Answer from the drawing. Dimensions are ordinates in mm from the lowest x, y and z of the part. A direction names the side the tool comes from. Coordinates: 2 decimals unless noted, no trailing zeros. Write each loop counter-clockwise with the first axis right and the second up, starting at its lowest first coordinate (ties: lowest second). Pieces come first, ordered by that corner, then holes.
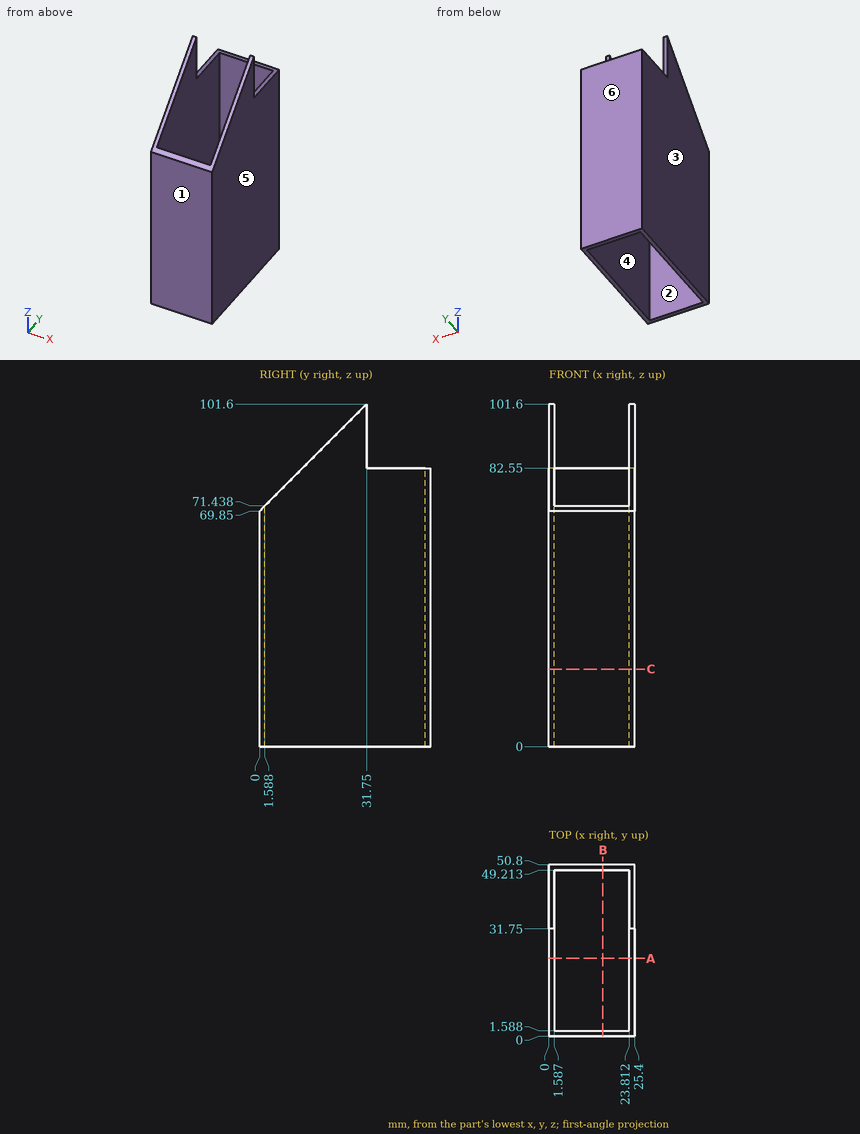
(1) This flat-tipped pin is pushed along its axis until it touches: pin 1 (0.5 mm diameter, centred on x = 25, z = 89.5, fed in from +Y). Where does it stop, or does it pass through?
(2) Which of the six approach directions +Z, -Z, +X, -X, +Y, -Y give full straight-line access (tool end or side, diameter ignored) to the marked faces 1 and 2?
(3) Find the intervals of material crossed by probe 1 along X at (y, z) = (39, 30.5); probe 2 along Y at (x, z) = (20, 25); probe 3 along Y at (x, z) = (18.75, 71.5), in increasing order.
(4) Section C-C, the plane z = 23 is taken. Write down the section's boundary in (x, y).
(5) Section A-A, the plane y = 23 is taken. Write down the section's boundary in (x, z).
(6) For a pull along X with two mould halves and no side action, classify the marked faces 3, 4, 5 and 6 as pulls with the +X half, pulls with the -X half, needs draft (parallel to the pull), parting line crosses it, or undercut.
(7) Section B-B, the plane x = 16 is taken. Write down the section's boundary in (y, z).
Solution:
1. pin 1: stops at y = 31.75
2. face 1: +Z, -Z, +X, -X, -Y
2. face 2: +Z, -Z
3. probe 1: x = 0 to 1.59, 23.81 to 25.4
3. probe 2: y = 0 to 1.59, 49.21 to 50.8
3. probe 3: y = 49.21 to 50.8
4. outline: (0, 0) - (25.4, 0) - (25.4, 50.8) - (0, 50.8) - close; hole (1.59, 1.59) - (23.81, 1.59) - (23.81, 49.21) - (1.59, 49.21) - close
5. outline: (0, 0) - (1.59, 0) - (1.59, 92.85) - (0, 92.85) - close; (23.81, 0) - (25.4, 0) - (25.4, 92.85) - (23.81, 92.85) - close
6. face 3: pulls with the -X half
6. face 4: undercut
6. face 5: pulls with the +X half
6. face 6: needs draft
7. outline: (0, 0) - (1.59, 0) - (1.59, 71.44) - (0, 69.85) - close; (49.21, 0) - (50.8, 0) - (50.8, 82.55) - (49.21, 82.55) - close
